Input: part model. Units: mm. Frame: model coordinates. A direction names the side the tool comes from. Round coordinates to 2 decimals unless told otherwise and drop trailing zeros. Order: outer loops, then holes, each group sorted by start corner. A loop starts at its lowest first (then second) coordinate and runs counter-clockwise, first axis right, second up. Notation, with made-up numbers: M -39,81.5 L -13,81.5 A12 ccw -13,88.5 Z; hole C 35,78 d5. An arc over 180 degrees is marked long. One line per question, with ' | ' between items.
```python
from build123d import *

# Parameters (mm, degrees)
SKETCH_1_W          = 45
SKETCH_1_H          = 35
SKETCH_1_R          = 1.6
EXTRUDE_1_DEPTH     = 15
SKETCH_2_W          = 5
SKETCH_2_H          = 25
CUT_EXTRUDE_2_DEPTH = 15


with BuildPart() as part:
    # 草图1 → 凸台-拉伸1 (new body)
    with BuildSketch(Plane.XY):
        with Locations((0, -1.5)):
            Rectangle(SKETCH_1_W, SKETCH_1_H)
        with Locations((-19, 10)):
            Circle(SKETCH_1_R, mode=Mode.SUBTRACT)
        with Locations((19, 10)):
            Circle(SKETCH_1_R, mode=Mode.SUBTRACT)
        with Locations((19, -10)):
            Circle(SKETCH_1_R, mode=Mode.SUBTRACT)
        with Locations((-19, -10)):
            Circle(SKETCH_1_R, mode=Mode.SUBTRACT)
    extrude(amount=EXTRUDE_1_DEPTH)

    # 草图2 → 切除-拉伸-薄壁2 (cut)
    with BuildSketch(Plane.XY):
        with Locations((0, -1.5)):
            Rectangle(SKETCH_2_W, SKETCH_2_H)
        with Locations((10, -1.5)):
            Rectangle(SKETCH_2_W, SKETCH_2_H)
        with Locations((-10, -1.5)):
            Rectangle(SKETCH_2_W, SKETCH_2_H)
    extrude(amount=CUT_EXTRUDE_2_DEPTH, mode=Mode.SUBTRACT)


solid = part.part
```
Item 1: Section query B-B, the plane x = -12. Return loops of the section in (y, z).
Report:
outline: M -19,0 L -14,0 L -14,15 L -19,15 Z; M 11,0 L 16,0 L 16,15 L 11,15 Z
Item 2: Mould query, pull axis X, two halves, no side actions, for faces 3 (the flat face through (0, 16, 7)), 4 (the flat face through (-22.5, -2, 7)), 5 (the flat face through (10, 11, 7)), 6 (the flat face through (-10, -14, 7)). Classes: +X half, -X half, draft (parallel to the pull), parting line (faces both ways), or undercut.
Report:
face 3: draft | face 4: -X half | face 5: undercut | face 6: undercut
Item 3: Section query A-A, the plane y = -10. Return loops of the section in (x, z).
Report:
outline: M -22.5,0 L -20.6,0 L -20.6,15 L -22.5,15 Z; M -17.4,0 L -12.5,0 L -12.5,15 L -17.4,15 Z; M -7.5,0 L -2.5,0 L -2.5,15 L -7.5,15 Z; M 2.5,0 L 7.5,0 L 7.5,15 L 2.5,15 Z; M 12.5,0 L 17.4,0 L 17.4,15 L 12.5,15 Z; M 20.6,0 L 22.5,0 L 22.5,15 L 20.6,15 Z
Item 4: Access query for faces 1 (the flat face through (0, -19, 7)), 2 (the flat face through (-10, 11, 7)). Directions: +Z, -Z, +X, -X, +Y, -Y. A direction counts if a zero-diameter tool reaches every point of the face in a straight line with its end or side. Return the directions, or none.
Report:
face 1: +Z, -Z, +X, -X, -Y | face 2: +Z, -Z
Item 5: Section query C-C, the plane z = 3.5. Return loops of the section in (x, y).
Report:
outline: M -22.5,-19 L 22.5,-19 L 22.5,16 L -22.5,16 Z; hole C -19,-10 d3.2; hole C -19,10 d3.2; hole M -12.5,-14 L -7.5,-14 L -7.5,11 L -12.5,11 Z; hole M -2.5,-14 L 2.5,-14 L 2.5,11 L -2.5,11 Z; hole M 7.5,-14 L 12.5,-14 L 12.5,11 L 7.5,11 Z; hole C 19,-10 d3.2; hole C 19,10 d3.2
Item 6: Section query D-D, the plane x = -19. Return loops of the section in (y, z).
Report:
outline: M -19,0 L -11.6,0 L -11.6,15 L -19,15 Z; M -8.4,0 L 8.4,0 L 8.4,15 L -8.4,15 Z; M 11.6,0 L 16,0 L 16,15 L 11.6,15 Z
Item 7: Line query: line 1 along X through (y, z) = (5, 3.5); line 2 along Y through (x, z) = (-19, 8.25); line 3 along Y through (x, z) = (10, 8.5). Output: solid intervals per line, ascending. Write a range as from..to.
Report:
line 1: -22.5..-12.5, -7.5..-2.5, 2.5..7.5, 12.5..22.5 | line 2: -19..-11.6, -8.4..8.4, 11.6..16 | line 3: -19..-14, 11..16
